from build123d import *

# Parameters (mm, degrees)
BOX_W           = 27
BOX_H           = 12
BOX_DEPTH       = 45
SKETCH_W        = 23
SKETCH_H        = 40
POCKET_DEPTH    = 10
SKETCH002_R     = 1
POCKET001_DEPTH = 5.001
SKETCH003_R     = 3
POCKET002_DEPTH = 3.5
SKETCH004_R     = 2.4
POCKET003_DEPTH = 2.001
PAD_DEPTH       = 2
FILLET_R        = 0.9
FILLET001_R     = 0.8


with BuildPart() as part:
    # Box → Box (new body)
    with BuildSketch(Plane.XY):
        with Locations((13.5, 6)):
            Rectangle(BOX_W, BOX_H)
    extrude(amount=BOX_DEPTH)

    # Sketch (on Face3 of BaseFeature) → Pocket (cut)
    with BuildSketch(Plane.XZ):
        with Locations((13.5, 20)):
            Rectangle(SKETCH_W, SKETCH_H)
    extrude(amount=-POCKET_DEPTH, mode=Mode.SUBTRACT)

    # Sketch002 (on Face7 of Pocket) → Pocket001 (cut, through all)
    with BuildSketch(Plane(origin=(0, 0, 40), x_dir=(1, 0, 0), z_dir=(0, 0, -1))):
        with Locations((13.5, -5)):
            Circle(SKETCH002_R)
    extrude(amount=-POCKET001_DEPTH, mode=Mode.SUBTRACT)

    # Sketch003 (on Face7 of Pocket001) → Pocket002 (cut)
    with BuildSketch(Plane(origin=(0, 0, 40), x_dir=(1, 0, 0), z_dir=(0, 0, -1))):
        with Locations((13.5, -5)):
            Circle(SKETCH003_R)
    extrude(amount=-POCKET002_DEPTH, mode=Mode.SUBTRACT)

    # Sketch004 (on Face11 of Pocket002) → Pocket003 (cut, through all)
    with BuildSketch(Plane.XZ.offset(-10)):
        with Locations((4.75, 6)):
            Circle(SKETCH004_R)
        with Locations((22.25, 6)):
            Circle(SKETCH004_R)
    extrude(amount=-POCKET003_DEPTH, mode=Mode.SUBTRACT)

    # Sketch006 (on Face3 of Pocket003) → Pad (join)
    with BuildSketch(Plane.XY.offset(45)):
        Polygon((3.4, 10.497498), (1.402502, 10.397498), (1.502502, 8.4), (3.5, 8.5), align=None)
        Polygon((1.502502, 3.6), (3.5, 3.5), (3.4, 1.502502), (1.402502, 1.602502), align=None)
        Polygon((23.5, 3.5), (25.497498, 3.6), (25.597498, 1.602502), (23.6, 1.502502), align=None)
        Polygon((23.6, 10.497498), (25.597498, 10.397498), (25.497498, 8.4), (23.5, 8.5), align=None)
    extrude(amount=PAD_DEPTH)

    # Fillet
    fillet_edges = [part.edges().sort_by_distance(p)[0] for p in [
        (27, 12, 22.5),
        (27, 6, 45),
        (13.5, 12, 45),
        (0, 6, 45),
        (0, 12, 22.5),
    ]]
    fillet(fillet_edges, radius=FILLET_R)

    # Fillet001
    fillet001_edges = [part.edges().sort_by_distance(p)[0] for p in [
        (2.401251, 1.552502, 47),
        (2.401251, 10.447498, 47),
        (24.598749, 10.447498, 47),
        (24.598749, 1.552502, 47),
    ]]
    fillet(fillet001_edges, radius=FILLET001_R)


solid = part.part
Verification items for the finished model (mm, model axes). A direction names the side the tool comes from. Round coordinates to 2 decimals unless told otherwise and drop trailing zeros. Loops run counter-clockwise (first coordinate to the right, second up) from the corner with the lowest first, then second, coordinate; pieces in that order, holes last. Notation, with made-up numbers: M -37.5,12.25 L -13.5,12.25 A26 ccw -13.5,37.25 Z; hole C 51,54 d4. An arc over 180 degrees is marked long. Write each question's results on one line, items separated by ' | '.
1) Scan lines: L1, parallel to X at y = 8.25, z = 11.5; L2, parallel to X at y = 5, z = 42.35; L3, parallel to Y at x = 13.5, z = 44.1. Record each from-to range of solid material in increasing order. Write a range as from..to.
Checks:
L1: x = 0..2, 25..27 | L2: x = 0..10.5, 16.5..27 | L3: y = 0..4, 6..12
2) Section check B-B on z = 6. Record the boundary of the cut face in (x, y), then the cut area to 3 significant figures.
Checks:
outline: M 0,0 L 2,0 L 2,10 L 2.35,10 L 2.35,12 L 0.9,12 A0.9 ccw 0,11.1 Z; M 7.15,10 L 19.85,10 L 19.85,12 L 7.15,12 Z; M 24.65,10 L 25,10 L 25,0 L 27,0 L 27,11.1 A0.9 ccw 26.1,12 L 24.65,12 Z | area: 74.5 mm2
3) Section check C-C on y = 5. Record the boundary of the cut face in (x, z).
Checks:
outline: M 0,0 L 2,0 L 2,40 L 10.5,40 L 10.5,43.5 L 12.5,43.5 L 12.5,45 L 0.9,45 A0.9 ccw 0,44.1 Z; M 14.5,43.5 L 16.5,43.5 L 16.5,40 L 25,40 L 25,0 L 27,0 L 27,44.1 A0.9 ccw 26.1,45 L 14.5,45 Z
4) Mould release check, pull along Z, two halves, no side actions. Record for faces 1 (the flat face through (24.613, 1.553, 45.592)), 2 (the flat face through (13, 11, 0)), 3 (the cylindrical face through (7.04, 10.99, 6.72)): released by +Z, released by -Z, zero draft, split by the parting line, or undercut.
Checks:
face 1: zero draft | face 2: released by -Z | face 3: undercut
5) Section check D-D on z = 42. Record the boundary of the cut face in (x, y), then the cut area to 3 significant figures.
Checks:
outline: M 0,0 L 27,0 L 27,11.1 A0.9 ccw 26.1,12 L 0.9,12 A0.9 ccw 0,11.1 Z; hole C 13.5,5 d6 | area: 295 mm2
6) Gauge pin test, flat ends, axial feed: P1, Ø4.5, axis at x = 4.75, z = 6, coming from the +Y side; P2, Ø5.5, axis at x = 11.5, y = 3, coming from the +Z side; P3, Ø5, axis at x = 14.5, y = 3.5, coming from the -Z side. Record the tip position at first contact, or that the pin passes through.
Checks:
P1: passes through | P2: stops at z = 45 | P3: stops at z = 40
7) Section check A-A on x = 22.25. Record the boundary of the cut face in (y, z), then the cut area to 3 significant figures.
Checks:
outline: M 0,40 L 10,40 L 10,8.4 L 12,8.4 L 12,44.1 A0.9 ccw 11.1,45 L 0,45 Z; M 10,0 L 12,0 L 12,3.6 L 10,3.6 Z | area: 130 mm2
8) Access from +Z, -Z, +X, -X, +Y, -Y to the whole of each face (thin tool, end or side, straight path). Record for faces 4 (the flat face through (2.49, 3.55, 45.99)), 5 (the flat face through (2.42, 1.55, 45.59)), 6 (the flat face through (23.55, 2.49, 45.99)).
Checks:
face 4: +Z | face 5: +Z, -X, -Y | face 6: +Z, -Y
